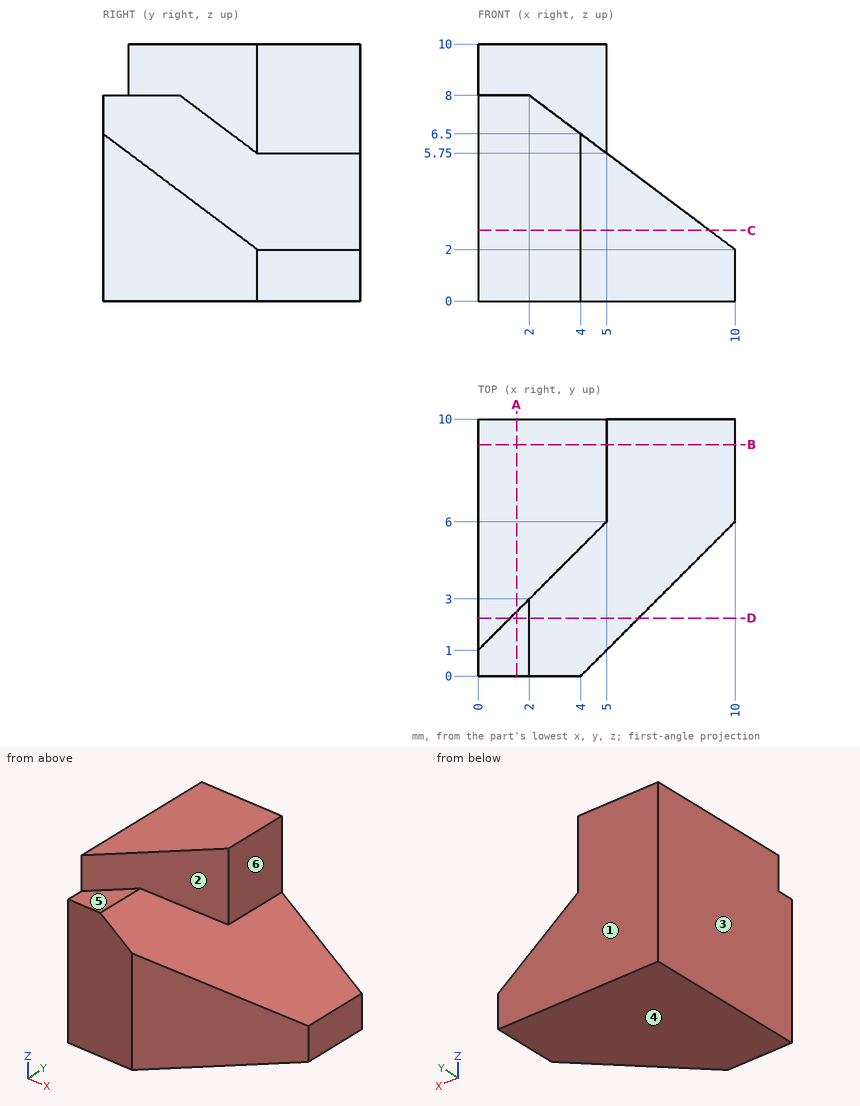
Design review of the part shown in the three views and the two pictorial views. Dimensions are in mm from the part's minimum x, y and z. A direction names the side the tool comes from. Coordinates: 2 decimals unless noted, no trailing zeros. Loops run counter-clockwise (first coordinate to the right, second up) from the corner with the lowest first, then second, coordinate; pieces in that order, holes last. Notation, with made-up numbers: (81, -18) - (124, -18) arc R17 ccw to (124, -4) - close; hole circle Ø10 at (-3.5, 35.5). An arc over 180 degrees is marked (long way). Use a Markdown table: item, result. Add a question column.
Item 1: We need section C-C (z = 2.75). Give the boundary of the cut face in (x, y).
Item 2: We need section D-D (y = 2.25). Give the boundary of the cut face in (x, z), and give its area (3 significant figures).
Item 3: We need section A-A (x = 1.5). Give the boundary of the cut face in (y, z), and give its area (3 significant figures).
Item 4: For line 1 (X direction, y = 8.5, z = 7.25); line 2 (X direction, y = 2, z = 8.25), list the stretches that pass through material, from the lowest coordinate up.
Item 5: Mouldability with a two-part tool opening along X and no side actions: class the marked faces 1, 2 and 3 as pulls with the +X half, pulls with the -X half, needs draft (parallel to the pull), parting line crosses it, or undercut.
Item 6: We need section B-B (y = 9). Give the boundary of the cut face in (x, z).
Item 7: Tool access review of the marked faces 4, 5 and 6: name each direction out of +Z, -Z, +X, -X, +Y, -Y from which nothing blocks a thin tool from reaching the whole face with its end or side.
Item 8: Insertion check: pin 1 Ø6 at (x, y) = (8, 3.5) entering from +Z; pin 2 Ø3 at (y, z) = (8, 7.5) entering from +X; pin 3 Ø4 at (y, z) = (9, 5) entering from +X; pin 4 Ø1 at (x, y) = (0.5, 1) entering from +Z. Each pin has a flat end and moves straight along its axis. Give the tip position at first contact, or say it passes through.
Results list:
| question | item | result |
|---|---|---|
| 1 | outline | (0, 0) - (4, 0) - (9, 5) - (9, 10) - (0, 10) - close |
| 2 | outline | (0, 0) - (6.25, 0) - (6.25, 4.81) - (2, 8) - (1.25, 8) - (1.25, 10) - (0, 10) - close |
| 2 | area | 45.7 mm^2 |
| 3 | outline | (0, 0) - (10, 0) - (10, 10) - (2.5, 10) - (2.5, 8) - (0, 8) - close |
| 3 | area | 95.0 mm^2 |
| 4 | line 1 | x = 0 to 5 |
| 4 | line 2 | x = 0 to 1 |
| 5 | face 1 | needs draft |
| 5 | face 2 | pulls with the +X half |
| 5 | face 3 | pulls with the -X half |
| 6 | outline | (0, 0) - (10, 0) - (10, 2) - (5, 5.75) - (5, 10) - (0, 10) - close |
| 7 | face 4 | -Z, +X, -X, +Y, -Y |
| 7 | face 5 | +Z, +X, -Y |
| 7 | face 6 | +Z, +X, +Y, -Y |
| 8 | pin 1 | stops at z = 5.75 |
| 8 | pin 2 | stops at x = 5 |
| 8 | pin 3 | stops at x = 8.67 |
| 8 | pin 4 | stops at z = 10 |
